The model under review builds one solid part; all positions refer to its coordinate system, in mm. Coordinates: 2 decimals unless noted, no trailing zeros. Order: outer loops, then holes, each group sorted by start corner. A loop starts at its lowest first (then second) coordinate and runs counter-clockwise, first axis right, second up. Notation, with made-up numbers: (5.5, 49) -> (58.5, 49) arc R18 cw to (58.5, 81) -> close; hole circle Ø7 at (89, -23). An arc over 180 degrees is marked (long way). Use CSV: the item, a comma, the result in double quotes. Start each with the question number.
Autodesk Inventor part; units mm, degrees
ref_plane "YZ Plane" through (0, 0, 0) normal (1, 0, 0) x (0, 1, 0)
ref_plane "XZ Plane" through (0, 0, 0) normal (0, 1, 0) x (-1, 0, 0)
ref_plane "Work Plane1" through (0, 0, 44.5407) normal (0, 0, 1) x (1, 0, 0)
sketch "Sketch2" plane through (0, 0, 44.5407) normal (0, 0, 1) x (1, 0, 0)
  line L0 (0, 34.026) -> (32.3607, 10.5146)
  line L1 (32.3607, 10.5146) -> (20, -27.5276)
  line L2 (20, -27.5276) -> (-20, -27.5276)
  line L3 (-20, -27.5276) -> (-32.3607, 10.5146)
  line L4 (-32.3607, 10.5146) -> (0, 34.026)
  point P0 (0, 0)
  point P1 (0, 0)
  dimension "d2" = 40
loft "Loft1" add profiles "Sketch2" section 2 point at (0, 0, 0)
mirror "Mirror1" about plane through (32.3607, 10.5146, 44.5407) normal (0.809017, -0.2628656, -0.5257311) of "Loft1"
mirror "Mirror2" about plane through (20, -27.5276, 44.5407) normal (0, -0.8506508, -0.5257311) of "Loft1"
mirror "Mirror3" about plane through (-20, -27.5276, 44.5407) normal (-0.809017, -0.2628656, -0.5257311) of "Loft1"
mirror "Mirror4" about plane through (-32.3607, 10.5146, 44.5407) normal (-0.5, 0.688191, -0.5257311) of "Loft1"
mirror "Mirror5" about plane through (0, 34.026, 44.5407) normal (0.5, 0.688191, -0.5257311) of "Loft1"
mirror "Mirror6" about plane through (-52.3607, -17.013, -10.5146) normal (0.309017, -0.4253254, -0.8506508) of "Loft1", "Mirror3"
mirror "Mirror7" about plane through (-52.3607, 17.013, 10.5146) normal (0, 0.5257311, -0.8506508) of "Loft1", "Mirror3"
mirror "Mirror8" about plane through (52.3607, -17.013, -10.5146) normal (0, 0.5257311, -0.8506508) of "Loft1", "Mirror1"
mirror "Mirror9" about plane through (20, 27.5276, -44.5407) normal (-0.809017, -0.2628656, -0.5257311) of "Loft1", "Mirror1", "Mirror8"
properties part number "dodecahedron"
Q1. Add section A-A, the plane z = -8. State the section outline as (x, y) points, then the cut area to 3 significant figures.
Q2. Clearance check with flat-ended pins moving along their axes: pin 1 Ø1 at (y, z) = (-40.5, -29) entering from +X; pin 2 Ø1 at (y, z) = (39.5, 27) entering from +X; pin 3 Ø12 at (x, z) = (40.5, -13) entering from -Y. State where each tip first meets the part, or that it passes through.
Q3. Add section C-C, the plane x = -3. State the section outline as (y, z) points.
Q4. To check wall thickness, follow probe 1 along X at (y, z) = (20, -25.5); probe 2 along Y at (x, z) = (-4, 24.5); probe 3 along X at (y, z) = (-10, 40.5). State the ranges of each line that lie inside material, in increasing order.
Q5. Add section D-D, the plane z = 18.5. State the section outline as (x, y) points.
Q6. Add section B-B, the plane y = 30. State the section outline as (x, z) points.
Answer block:
1,outline,"(-52.36, -12.94) -> (-49.97, -20.3) -> (-3.87, -53.8) -> (3.87, -53.8) -> (49.97, -20.3) -> (52.36, -12.94) -> (34.75, 41.25) -> (28.49, 45.8) -> (-28.49, 45.8) -> (-34.75, 41.25) -> close"
1,area,"7,570 mm²"
2,pin 1,"stops at x = 5.12"
2,pin 2,"stops at x = 8.2"
2,pin 3,"stops at y = -29.82"
3,outline,"(-54.08, -8.57) -> (-31.85, -44.54) -> (27.53, -44.54) -> (54.08, 8.57) -> (31.85, 44.54) -> (-27.53, 44.54) -> close"
4,probe 1,"x = -32.46 to 32.46"
4,probe 2,"y = -37.55 to 43.51"
4,probe 3,"x = -27.82 to 27.82"
5,outline,"(-47.67, 15.49) -> (-29.46, -40.55) -> (29.46, -40.55) -> (47.67, 15.49) -> (0, 50.12) -> close"
6,outline,"(-42.93, 0.59) -> (-21.8, -39.6) -> (21.8, -39.6) -> (42.93, 0.59) -> (5.54, 44.54) -> (-5.54, 44.54) -> close"
